Part print with two shaded views. Sizes in mm from the minimum x, y, z corner. A direction names the side the tool comes from. Coordinates: 2 decimals unless noted, no trailing zeros. Loops run counter-clockwise (first coordinate to the right, second up) from the corner with the lowest first, then second, coordinate; pieces in that order, holes last. Notation, with made-up numbers: (-15.5, 72.25) -> (0.5, 72.25) arc R21 ccw to (0.5, 76.25) -> close; hole circle Ø2 at (35.5, 32). An arc over 180 degrees is marked (long way). Answer as a JSON object with one key per item and string values. Group by question number.
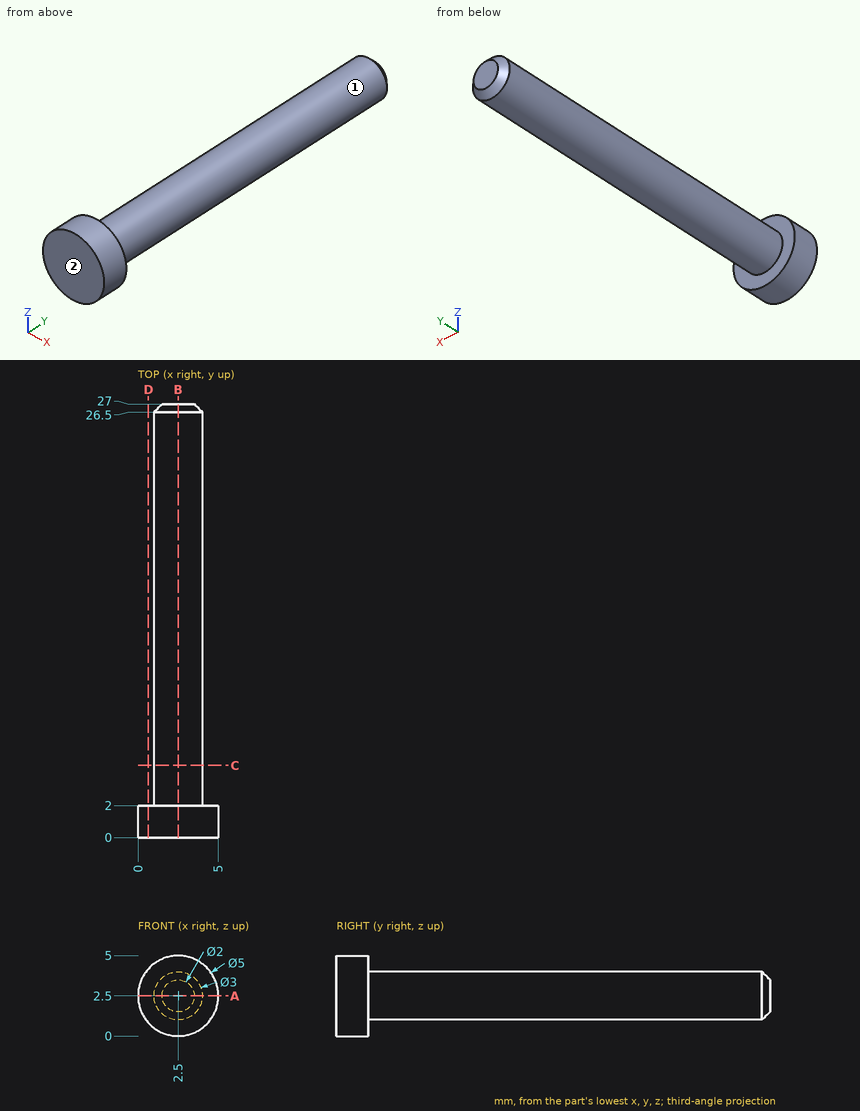
Item 1: Drill centre lines: L1, parallel to Y at x = 4.5, z = 1.35; L2, parallel to X at y = 9, z = 2.55; L3, parallel to Z at x = 1.3, y = 25.25. Where is each one in solid material? Low to high.
Item 2: 3-axis set-ups, long thin cutter, end or side, ignore diameter. For the marked faces 1 and 2: which of +Z, -Z, +X, -X, +Y, -Y reach the whole face in a straight line?
Item 3: Band-saw the part on A-A, the plane z = 2.5. List the corners of the cut face in (x, y), and give its area (4 significant figures).
Item 4: Flat gauge pins, fed straight in: P1, Ø3, axis at x = 2, y = 16, coming from the -Z side; P2, Ø2, axis at y = 24, z = 3.5, coming from the +X side; P3, Ø2, axis at x = 0.5, z = 0.5, coming from the -Y side. Where does each tip first touch, or does it go through?
Item 5: Band-saw the part on C-C, the plane y = 4.5. List the corners of the cut face in (x, z), and give its area (3 significant figures).
Item 6: Band-saw the part on D-D, the plane x = 0.65. List the corners of the cut face in (y, z).
Item 7: Band-saw the part on B-B, the plane x = 2.5. List the corners of the cut face in (y, z).
Reply:
{
 "1": {"L1": "0 to 2", "L2": "1 to 4", "L3": "1.6 to 3.4"},
 "2": {"face 1": "+Y", "face 2": "+Z, -Z, +X, -X, -Y"},
 "3": {"outline": "(0, 0) -> (5, 0) -> (5, 2) -> (4, 2) -> (4, 26.5) -> (3.5, 27) -> (1.5, 27) -> (1, 26.5) -> (1, 2) -> (0, 2) -> close", "area": "84.75 mm²"},
 "4": {"P1": "z = 1", "P2": "x = 4", "P3": "y = 0"},
 "5": {"outline": "circle Ø3 at (2.5, 2.5)", "area": "7.07 mm²"},
 "6": {"outline": "(0, 0.82) -> (2, 0.82) -> (2, 4.18) -> (0, 4.18) -> close"},
 "7": {"outline": "(0, 0) -> (2, 0) -> (2, 1) -> (26.5, 1) -> (27, 1.5) -> (27, 3.5) -> (26.5, 4) -> (2, 4) -> (2, 5) -> (0, 5) -> close"}
}
